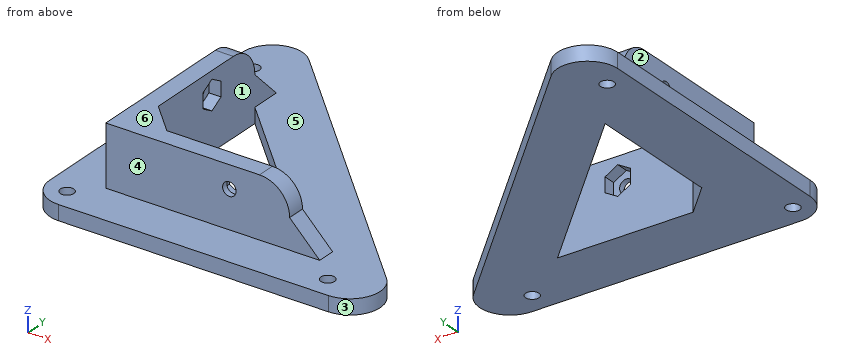
```python
from build123d import *

# Parameters (mm, degrees)
F0_R      = 2.25
F1_DEPTH  = 5
F3_DEPTH  = 20
F4_R      = 10
F5_R      = 2.25
F6_DEPTH  = 25
F7_R      = 2.25
F8_DEPTH  = 25
F9_SIZE   = 9.99999
F11_DEPTH = 4
F13_DEPTH = 4


# Not quite as in the source:
# - a fillet or chamfer is up to 0.001 mm smaller than in the source, because OpenCascade refuses the exact size


with BuildPart() as f1:
    # F0 (on Top) → F1 (new body)
    with BuildSketch(Plane.XY):
        Polygon((123.7436867076, 0), (0, 123.7436867076), (0, 103.7436867076), (0, 0), (103.7436867076, 0), align=None)
        with Locations((7.5, 7.5)):
            Circle(F0_R, mode=Mode.SUBTRACT)
        Polygon((21, 21), (21, 76), (76, 21), align=None, mode=Mode.SUBTRACT)
        with Locations((94, 7.5)):
            Circle(F0_R, mode=Mode.SUBTRACT)
        with Locations((7.5, 94)):
            Circle(F0_R, mode=Mode.SUBTRACT)
    extrude(amount=F1_DEPTH)

    # F2 (on face) → F3 (join)
    with BuildSketch(Plane.XY.offset(5)):
        Polygon((76, 15), (76, 21), (21, 21), (21, 76), (15, 76), (15, 15), align=None)
    extrude(amount=F3_DEPTH)

    # F4
    f4_edges = [f1.edges().sort_by_distance(p)[0] for p in [
        (0, 123.743687, 2.5),
        (123.743687, 0, 2.5),
        (76, 18, 25),
        (18, 76, 25),
        (0, 0, 2.5),
    ]]
    fillet(f4_edges, radius=F4_R)

    # F5 (on face) → F6 (cut)
    with BuildSketch(Plane.YZ.offset(21)):
        with Locations((56, 17.5)):
            Circle(F5_R)
    extrude(amount=-F6_DEPTH, mode=Mode.SUBTRACT)

    # F7 (on face) → F8 (cut)
    with BuildSketch(Plane(origin=(0, 21, 0), x_dir=(-1, 0, 0), z_dir=(0, 1, 0))):
        with Locations((-56, 17.5)):
            Circle(F7_R)
    extrude(amount=-F8_DEPTH, mode=Mode.SUBTRACT)

    # F9 (size 10 in the source; OpenCascade refuses exactly that, so slightly less here)
    f9_edges = [f1.edges().sort_by_distance(p)[0] for p in [
        (18, 76, 5),
        (76, 18, 5),
        (21, 21, 12.5),
    ]]
    chamfer(f9_edges, length=F9_SIZE)

    # F10 (on face) → F11 (cut)
    with BuildSketch(Plane(origin=(0, 21, 0), x_dir=(-1, 0, 0), z_dir=(0, 1, 0))):
        Polygon((-51.775, 15.0606951127), (-51.775, 19.9393048873), (-56, 22.3786097747), (-60.225, 19.9393048873), (-60.225, 15.0606951127), (-56, 12.6213902253), align=None)
    extrude(amount=-F11_DEPTH, mode=Mode.SUBTRACT)

    # F12 (on face) → F13 (cut)
    with BuildSketch(Plane.YZ.offset(21)):
        Polygon((60.225, 15.0606951127), (60.225, 19.9393048873), (56, 22.3786097747), (51.775, 19.9393048873), (51.775, 15.0606951127), (56, 12.6213902253), align=None)
    extrude(amount=-F13_DEPTH, mode=Mode.SUBTRACT)


solid = f1.part
```
The listing builds one solid part. Answer for the finished solid, in the listing's coordinates (mm). Face numbers are marked on the shaded views. A direction names the side the tool comes from. Coordinates: 2 decimals unless noted, no trailing zeros. Write each loop counter-clockwise with the first axis right and the second up, starting at its lowest first coordinate (ties: lowest second). Pieces come first, ordered by that corner, then holes. Notation, with made-up numbers: M 61.25,-15.5 L 110.25,-15.5 A17 cw 110.25,-8.5 Z; hole C 68.25,39 d4. An arc over 180 degrees is marked long. Use a Markdown table: item, result. Add a question column.
1. Section C-C (z = 17.5) is taken. Give the vertices of the cut face in (x, y) (3 decimals).
2. Given P1, Ø6, axis at y = 49, z = 11, coming from the -X side; P2, Ø2, axis at y = 15.5, z = 9, coming from the +X side; P3, Ø6, axis at x = 94, y = 7.5, coming from the +Z side, each flat-ended and moving along its own axis, determine where each tip first touches the part or whether it passes through.
3. Straight lines are drawn through the part: line 1 along Y through (x, z) = (7.5, 2.5); line 2 along X through (y, z) = (78, 11.75); line 3 along Z through (x, y) = (22, 81). For each, find the intervals that lie inside material, in ascending order. Write a range as [from, to].
4. Section D-D (y = 67.5) is taken. Give the vertices of the cut face in (x, z), plus the area to 3 significant figures.
5. For a pull along X with two mould halves and no side action, classify the marked faces 1, 2 and 3 as +X half, -X half, draft (parallel to the pull), parting line (faces both ways), or undercut.
6. Section A-A (y = 7.5) is taken. Give the vertices of the cut face in (x, z), plus the area to 3 significant figures.
7. Which of the six approach directions +Z, -Z, +X, -X, +Y, -Y give full straight-line access (tool end or side, diameter ignored) to the marked faces 4, 5 and 6?
Data:
| question | item | result |
|---|---|---|
| 1 | outline | M 15,15 L 53.75,15 L 53.75,17 L 51.775,17 L 51.775,21 L 31,21 L 21,31 L 21,51.775 L 17,51.775 L 17,53.75 L 15,53.75 Z; M 15,58.25 L 17,58.25 L 17,60.225 L 21,60.225 L 21,75.682 L 15,75.682 Z; M 58.25,15 L 75.682,15 L 75.682,21 L 60.225,21 L 60.225,17 L 58.25,17 Z |
| 2 | P1 | stops at x = 15 |
| 2 | P2 | stops at x = 83 |
| 2 | P3 | stops at z = 5 |
| 3 | line 1 | y = [0.32, 5.25], [9.75, 91.75], [96.25, 109.28] |
| 3 | line 2 | x = [15, 21] |
| 3 | line 3 | z = [0, 5] |
| 4 | outline | M 0,0 L 21,0 L 21,24.89 L 15,24.89 L 15,5 L 0,5 Z; M 29.5,0 L 56.24,0 L 56.24,5 L 29.5,5 Z |
| 4 | area | 358 mm2 |
| 5 | face 1 | undercut |
| 5 | face 2 | -X half |
| 5 | face 3 | +X half |
| 6 | outline | M 0.32,0 L 5.25,0 L 5.25,5 L 0.32,5 Z; M 9.75,0 L 91.75,0 L 91.75,5 L 9.75,5 Z; M 96.25,0 L 109.28,0 L 109.28,5 L 96.25,5 Z |
| 6 | area | 500 mm2 |
| 7 | face 4 | +Z, +X, -X, -Y |
| 7 | face 5 | +Z |
| 7 | face 6 | +Z, +X, -X, +Y, -Y |
